Verification items for the finished model (mm, model axes). Face numbers are marked on the shaded views. A direction names the side the tool comes from. Round coordinates to 2 decimals unless told otherwise and drop trailing zeros. Write each loop counter-clockwise with the first axis right and the second up, starting at its lowest first coordinate (ties: lowest second). Pieces come first, ordered by that corner, then holes. Notation, with made-up numbers: (75, 34.5) -> (117, 34.5) arc R33 ccw to (117, 62.5) -> close; hole circle Ø9 at (28, -25.75). An arc over 180 degrees is marked (long way). Answer as a JSON object with one key per item and string values. Group by question number.
(1) Sectioned sample at D-D on z = -9. Count the separate pieces of the cut face and the enclosed holes in it, and give its area (3 significant figures).
(2) Sectioned sample at C-C on z = 18. Record the cut outline in (x, y).
(3) Draft check along Z on the marked faces 4, 5 and 6. Enter one of: released by +Z, released by -Z, zero draft, split by the parting line, or undercut.
(4) Sectioned sample at B-B on y = 8.5. Record the cut outline in (x, z).
(5) Scan lines: L1, parallel to Z at x = 0, y = -18.35; L2, parallel to Z at x = 0, y = 8; L3, parallel to X at y = -19, z = 0. Record each from-to range of solid material in increasing order. Write a range as from..to.
(6) Gauge pin test, flat ends, axial feed: pin 1 Ø4 at (x, y) = (-4, -6) entering from +Z; pin 2 Ø8 at (y, z) = (-13, 14.5) entering from +X; pin 3 Ø11.5 at (x, z) = (0, 0) entering from +Y; pin 4 Ø12 at (y, z) = (7, 7) entering from -X. Record the tip position at first contact, or that the pin passes through.
(7) Set-up check for the marked faces 1, 2 and 3: record each of +Z, -Z, +X, -X, +Y, -Y from which the full face is reachable in a straight line by a thin tool's end or side.
(8) Sectioned sample at A-A on z = 0. Record the cut outline in (x, y).
```python
from build123d import *

# Parameters (mm, degrees)
F2_SIZE = 1
F4_D    = 3.3


with BuildPart() as f1:
    # F0 (on Right) → F1 (revolve)
    with BuildSketch(Plane.YZ):
        Polygon((-15.9130460173, 6.5), (18.0869539827, 6.5), (18.0869539827, 11.5), (-8.9130460173, 11.5), (-8.9130460173, 23), (-21.9130460173, 23), (-21.9130460173, 13), (-15.9130460173, 13), align=None)
    revolve(axis=Axis((0, -2.1911122165, 0), (0, -1, 0)))

    # F2
    f2_edges = [f1.edges().sort_by_distance(p)[0] for p in [
        (0, 18.086954, -11.5),
        (0, 18.086954, -6.5),
        (0, -21.913046, -13),
    ]]
    chamfer(f2_edges, length=F2_SIZE)

    # F4 (through all)
    with Locations(Plane.XZ.offset(21.9130460173)):
        with Locations((0, 18), (-15.5884572681, -9), (15.5884572681, -9)):
            Hole(F4_D / 2)


solid = f1.part
```
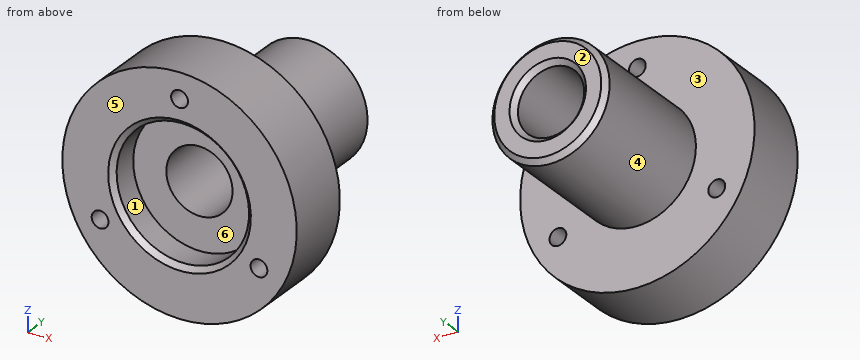
Computed values:
{
 "1": {"separate pieces": "3", "enclosed holes": "0", "area": "735 mm2"},
 "2": {"outline": "(-14.32, -21.91) -> (-1.65, -21.91) -> (-1.65, -8.91) -> (-14.32, -8.91) -> close; (1.65, -21.91) -> (14.32, -21.91) -> (14.32, -8.91) -> (1.65, -8.91) -> close"},
 "3": {"face 4": "split by the parting line", "face 5": "zero draft", "face 6": "undercut"},
 "4": {"outline": "circle Ø23 at (0, 0); hole circle Ø13 at (0, 0)"},
 "5": {"L1": "-23..-13, 13..16.35, 19.65..23", "L2": "-11.5..-6.5, 6.5..11.5", "L3": "-23..-13, 13..23"},
 "6": {"pin 1": "z = 11.32", "pin 2": "x = 20.46", "pin 3": "through", "pin 4": "x = -11.46"},
 "7": {"face 1": "-Y", "face 2": "+Z, -Z, +X, -X, +Y", "face 3": "+Y"},
 "8": {"outline": "(-23, -21.91) -> (-14, -21.91) -> (-13, -20.91) -> (-13, -15.91) -> (-6.5, -15.91) -> (-6.5, 17.09) -> (-7.5, 18.09) -> (-10.5, 18.09) -> (-11.5, 17.09) -> (-11.5, -8.91) -> (-23, -8.91) -> close; (6.5, -15.91) -> (13, -15.91) -> (13, -20.91) -> (14, -21.91) -> (23, -21.91) -> (23, -8.91) -> (11.5, -8.91) -> (11.5, 17.09) -> (10.5, 18.09) -> (7.5, 18.09) -> (6.5, 17.09) -> close"}
}
